The listing builds one solid part. Answer for the finished solid, in the listing's coordinates (mm). A direction names the side the tool comes from. Coordinates: 2 decimals unless noted, no trailing zeros. Order: outer loops, then holes, each group sorted by start corner. A loop starts at its lowest first (then second) coordinate and runs counter-clockwise, first axis right, second up. Notation, with made-up numbers: (1.5, 24.25) -> (56.5, 24.25) arc R31 ccw to (56.5, 59.25) -> close; hole circle Ø3 at (80, 22). An arc over 180 degrees is marked (long way). Return JSON: item names as keys, results as strings.
from build123d import *

# Parameters (mm, degrees)
CROQUIS1_W               = 108
CROQUIS1_H               = 71
SALIENTE_EXTRUIR1_DEPTH  = 1.5
CROQUIS2_W               = 12
CROQUIS2_H               = 3
CROQUIS2_W_2             = 8
CORTAR_EXTRUIR1_DEPTH    = 3
CROQUIS4_W               = 8
CROQUIS4_H               = 3
SALIENTE_EXTRUIR2_DEPTH  = 3
REDONDEO1_R              = 3
CROQUIS5_R               = 1.5
CORTAR_EXTRUIR2_DEPTH    = 13
REDONDEO1_OF_SIMETR_A2_R = 3
CROQUIS6_W               = 3
CROQUIS6_H               = 14
CROQUIS6_H_2             = 8
CORTAR_EXTRUIR3_DEPTH    = 3
CROQUIS7_W               = 3.217414859
CROQUIS7_H               = 7.6
CORTAR_EXTRUIR4_DEPTH    = 73
CROQUIS8_R               = 6.5
CROQUIS8_R_2             = 3
CROQUIS8_R_3             = 1.5
CROQUIS8_W               = 3.259373519
CROQUIS8_H               = 6.723882433
CORTAR_EXTRUIR5_DEPTH    = 23


with BuildPart() as part:
    # Croquis1 → Saliente-Extruir1 (new, symmetric)
    with BuildSketch(Plane(origin=(0, 0, 0), x_dir=(0, 0, -1), z_dir=(1, 0, 0))):
        Rectangle(CROQUIS1_W, CROQUIS1_H)
    extrude(amount=SALIENTE_EXTRUIR1_DEPTH, both=True)

    # Croquis2 → Cortar-Extruir1 (cut)
    with BuildSketch(Plane.ZY.offset(1.5)):
        with Locations((-48, -34)):
            Rectangle(CROQUIS2_W, CROQUIS2_H)
        with Locations((-24, -34)):
            Rectangle(CROQUIS2_W_2, CROQUIS2_H)
        with Locations((-8, -34)):
            Rectangle(CROQUIS2_W_2, CROQUIS2_H)
        with Locations((8, -34)):
            Rectangle(CROQUIS2_W_2, CROQUIS2_H)
        with Locations((24, -34)):
            Rectangle(CROQUIS2_W_2, CROQUIS2_H)
        with Locations((48, -34)):
            Rectangle(CROQUIS2_W, CROQUIS2_H)
        with Locations((48, 34)):
            Rectangle(CROQUIS2_W, CROQUIS2_H)
        with Locations((24, 34)):
            Rectangle(CROQUIS2_W_2, CROQUIS2_H)
        with Locations((8, 34)):
            Rectangle(CROQUIS2_W_2, CROQUIS2_H)
        with Locations((-8, 34)):
            Rectangle(CROQUIS2_W_2, CROQUIS2_H)
        with Locations((-24, 34)):
            Rectangle(CROQUIS2_W_2, CROQUIS2_H)
        with Locations((-48, 34)):
            Rectangle(CROQUIS2_W, CROQUIS2_H)
    extrude(amount=-CORTAR_EXTRUIR1_DEPTH, mode=Mode.SUBTRACT)

    # Croquis4 → Saliente-Extruir2 (add)
    with BuildSketch(Plane.ZY.offset(1.5)):
        with Locations((16, 37)):
            Rectangle(CROQUIS4_W, CROQUIS4_H)
    saliente_extruir2 = extrude(amount=-SALIENTE_EXTRUIR2_DEPTH)

    # Redondeo1
    redondeo1_edges = [part.edges().sort_by_distance(p)[0] for p in [
        (0, 38.5, 12),
        (0, 38.5, 20),
    ]]
    fillet(redondeo1_edges, radius=REDONDEO1_R)

    # Croquis5 → Cortar-Extruir2 (cut)
    with BuildSketch(Plane.ZY.offset(1.5)):
        with Locations((16, 34)):
            Circle(CROQUIS5_R)
    cortar_extruir2 = extrude(amount=-CORTAR_EXTRUIR2_DEPTH, mode=Mode.SUBTRACT)

    # Simetr_a2: Saliente-Extruir2, Cortar-Extruir2 across plane
    add(saliente_extruir2.mirror(Plane.ZX))
    add(cortar_extruir2.mirror(Plane.ZX), mode=Mode.SUBTRACT)

    # Redondeo1 of Simetr_a2
    redondeo1_of_simetr_a2_edges = [part.edges().sort_by_distance(p)[0] for p in [
        (0, -38.5, 12),
        (0, -38.5, 20),
    ]]
    fillet(redondeo1_of_simetr_a2_edges, radius=REDONDEO1_OF_SIMETR_A2_R)

    # Croquis6 → Cortar-Extruir3 (cut)
    with BuildSketch(Plane.ZY.offset(1.5)):
        with Locations((52.5, -28.5)):
            Rectangle(CROQUIS6_W, CROQUIS6_H)
        with Locations((52.5, -6.5)):
            Rectangle(CROQUIS6_W, CROQUIS6_H_2)
        with Locations((52.5, 6.5)):
            Rectangle(CROQUIS6_W, CROQUIS6_H_2)
        with Locations((52.5, 28.5)):
            Rectangle(CROQUIS6_W, CROQUIS6_H)
    extrude(amount=-CORTAR_EXTRUIR3_DEPTH, mode=Mode.SUBTRACT)

    # Croquis7 → Cortar-Extruir4 (cut)
    with BuildSketch(Plane(origin=(0, 32.5, 0), x_dir=(1, 0, 0), z_dir=(0, 1, 0))):
        with Locations((-0.10870743, 50.2)):
            Rectangle(CROQUIS7_W, CROQUIS7_H)
    extrude(amount=-CORTAR_EXTRUIR4_DEPTH, mode=Mode.SUBTRACT)

    # Croquis8 → Cortar-Extruir5 (cut)
    with BuildSketch(Plane(origin=(1.5, 0, 0), x_dir=(0, 0, -1), z_dir=(1, 0, 0))):
        with Locations((23.8, -20.25)):
            Circle(CROQUIS8_R)
        with Locations((13, -20.25)):
            Circle(CROQUIS8_R_2)
        with Locations((3.2, -11.5)):
            Circle(CROQUIS8_R_3)
        with Locations((3.2, -29)):
            Circle(CROQUIS8_R_3)
        with Locations((-8.36450747, -20.229697644)):
            Rectangle(CROQUIS8_W, CROQUIS8_H)
    extrude(amount=-CORTAR_EXTRUIR5_DEPTH, mode=Mode.SUBTRACT)


solid = part.part
1. The part is cut by section D-D on x = 0.65. Give the number of separate pieces and of enclosed holes in the cut face, and give its area (3 significant figures).
Answer block:
{"separate pieces": "1", "enclosed holes": "7", "area": "6,550 mm2"}
2. The part is cut by section A-A on y = -34. Give the vertices of the cut face in (x, z).
Answer block:
{"outline": "(-1.5, -42) -> (1.5, -42) -> (1.5, -28) -> (-1.5, -28) -> close; (-1.5, -20) -> (1.5, -20) -> (1.5, -12) -> (-1.5, -12) -> close; (-1.5, -4) -> (1.5, -4) -> (1.5, 4) -> (-1.5, 4) -> close; (-1.5, 12) -> (1.5, 12) -> (1.5, 14.5) -> (-1.5, 14.5) -> close; (-1.5, 17.5) -> (1.5, 17.5) -> (1.5, 20) -> (-1.5, 20) -> close; (-1.5, 28) -> (1.5, 28) -> (1.5, 42) -> (-1.5, 42) -> close"}
3. The part is cut by section B-B on y = -20.25. Give the vertices of the cut face in (x, z), and give its area (3 significant figures).
Answer block:
{"outline": "(-1.5, -46.4) -> (1.5, -46.4) -> (1.5, -30.3) -> (-1.5, -30.3) -> close; (-1.5, -17.3) -> (1.5, -17.3) -> (1.5, -16) -> (-1.5, -16) -> close; (-1.5, -10) -> (1.5, -10) -> (1.5, 6.73) -> (-1.5, 6.73) -> close; (-1.5, 9.99) -> (1.5, 9.99) -> (1.5, 54) -> (-1.5, 54) -> close", "area": "234 mm2"}
4. For faces 1 (the face through (0, 2.5, 52)), 2 (the face through (0, -20, 9.994)), 3 (the face through (0, -34, -20)), 4 (the face through (0, 32.5, -24)), 5 (the face through (0, -35.5, -16)), determine the directions among +Z, -Z, +X, -X, +Y, -Y from which every point of the face is accessible in a straight line to the end or side of a thin tool.
Answer block:
{"face 1": "+Z, +X, -X", "face 2": "+X, -X", "face 3": "+X, -X, -Y", "face 4": "+X, -X, +Y", "face 5": "-Z, +X, -X, -Y"}
5. Consider line 1 (Z direction, x = -0.5, y = -34); line 2 (Y direction, x = 0.4, z = -3.2); line 3 (Y direction, x = 1.15, z = 35). Determine where each line is inside the solid, lowest interval first. Write a range as from..to.
Answer block:
{"line 1": "z = -42..-28, -20..-12, -4..4, 12..14.5, 17.5..20, 28..42", "line 2": "y = -35.5..-30.5, -27.5..-13, -10..35.5", "line 3": "y = -35.5..35.5"}
6. The part is cut by section C-C on z = -18.5. Give the vertices of the cut face in (x, y).
Answer block:
{"outline": "(-1.5, -35.5) -> (1.5, -35.5) -> (1.5, -24.01) -> (-1.5, -24.01) -> close; (-1.5, -16.49) -> (1.5, -16.49) -> (1.5, 35.5) -> (-1.5, 35.5) -> close"}
7. Each of these flat-tipped pins is pushed along its axis until it touches: pin 1 Ø1.5 at (x, y) = (-0.5, 7) entering from +Z; pin 2 Ø1.5 at (x, y) = (0.5, 34.5) entering from +Z; pin 3 Ø1.5 at (x, y) = (-0.5, -34) entering from -Z; pin 4 Ø1.8 at (y, z) = (-29, -3.2) entering from +X. Where does it stop, or does it pass through?
Answer block:
{"pin 1": "stops at z = 51", "pin 2": "stops at z = 42", "pin 3": "stops at z = -42", "pin 4": "passes through"}
8. Determine the mould class of faces 6 (the face through (0, -38.5, 16)), 7 (the face through (0, 34, 4)), 8 (the face through (0.02, 37.6, 19.14)) for opening direction Z: pulls with the +Z half, pulls with the -Z half, needs draft (parallel to the pull), parting line crosses it, or undercut.
Answer block:
{"face 6": "needs draft", "face 7": "undercut", "face 8": "pulls with the +Z half"}
